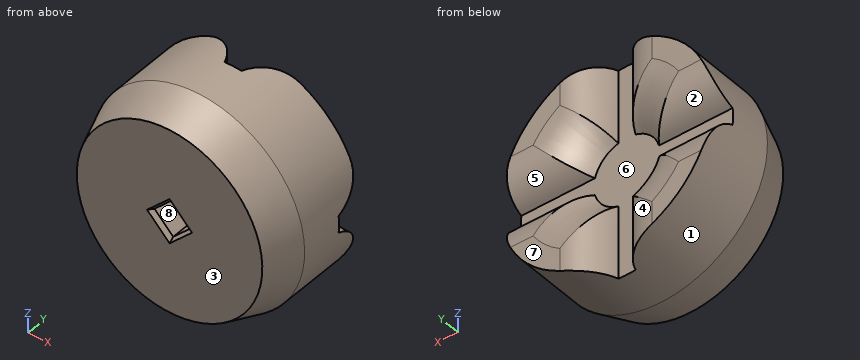
from build123d import *

# Parameters (mm, degrees)
SKETCH3_R           = 8
BOSS_EXTRUDE3_DEPTH = 8
CUT_EXTRUDE2_DEPTH  = 2
CUT_EXTRUDE2_DRAFT  = -10
SKETCH7_R           = 2.5
CUT_EXTRUDE4_DEPTH  = 2
FILLET1_R           = 5
FILLET2_START       = -9
FILLET2_DEPTH       = 18
FILLET2_2_DEPTH     = 18
CUT_EXTRUDE5_DEPTH  = 2.2
CHAMFER2_SIZE       = 0.2
CHAMFER2_SIZE2      = 0.346410162
CHAMFER3_SIZE       = 1
CHAMFER3_SIZE2      = 2.747477419


with BuildPart() as part:
    # Sketch3 → Boss-Extrude3 (new body)
    with BuildSketch(Plane(origin=(0, 0, 0), x_dir=(1, 0, 0), z_dir=(0, 1, 0))):
        with Locations(Location((0, 0, 0), (0, 0, 270))):
            Circle(SKETCH3_R)
    extrude(amount=BOSS_EXTRUDE3_DEPTH)


with BuildPart() as cut_extrude2_tool:
    # Sketch4 → Cut-Extrude2 (with draft: the straight prism first)
    with BuildSketch(Plane(origin=(0, 8, 0), x_dir=(1, 0, 0), z_dir=(0, 1, 0))):
        Polygon((-9, -1), (-1, -1), (-1, -9), (1, -9), (1, -1), (9, -1), (9, 1), (1, 1), (1, 9), (-1, 9), (-1, 1), (-9, 1), align=None)
    extrude(amount=-CUT_EXTRUDE2_DEPTH)
    # Cut-Extrude2: the draft: its side faces are tilted about the plane it starts from
    cut_extrude2_sides = [cut_extrude2_tool.faces().sort_by_distance(p)[0] for p in [
        (-5, 7, 1),
        (-1, 7, 5),
        (0, 7, 9),
        (1, 7, 5),
        (5, 7, 1),
        (9, 7, 0),
        (5, 7, -1),
        (1, 7, -5),
        (0, 7, -9),
        (-1, 7, -5),
        (-5, 7, -1),
        (-9, 7, 0),
    ]]
    draft(cut_extrude2_sides, Plane(origin=(0, 8, 0), x_dir=(1, 0, 0), z_dir=(0, 1, 0)), CUT_EXTRUDE2_DRAFT)


with BuildPart() as part_1:
    add(part.part)

    # Cut-Extrude2: cut by cut_extrude2_tool
    add(cut_extrude2_tool.part, mode=Mode.SUBTRACT)

    # Sketch7 → Cut-Extrude4 (cut)
    with BuildSketch(Plane(origin=(0, 8, 0), x_dir=(1, 0, 0), z_dir=(0, 1, 0))):
        Circle(SKETCH7_R)
    extrude(amount=-CUT_EXTRUDE4_DEPTH, mode=Mode.SUBTRACT)

    # Fillet1
    # the kernel refuses this fillet: 5 mm, written as the material it takes off along each edge
    with BuildSketch(Plane(origin=(0, 8, 0), x_dir=(-0.7093247295722765, 0, -0.7048818539423588), z_dir=(0.7048818539423588, 0, -0.7093247295722765))) as fillet1_piece_1:
        with BuildLine():
            CenterArc((6.5, -5), FILLET1_R, 90, 53.130102354)
            Line((2.5, -2), (2.42, -1.94))
            ThreePointArc((2.42, -1.94), (2.4, -1), (2.4, 0))
            Line((2.4, 0), (2.5, 0.1))
            Line((2.5, 0.1), (6.5, 0.1))
            Line((6.5, 0.1), (6.5, 0))
        make_face()
    revolve(axis=Axis((0, 8, 0), (0, 1, 0)), revolution_arc=359.64, mode=Mode.SUBTRACT)
    with BuildSketch(Plane(origin=(0, 8, 0), x_dir=(0.7048818539423484, 0, -0.7093247295722869), z_dir=(0.7093247295722869, 0, 0.7048818539423484))) as fillet1_piece_2:
        with BuildLine():
            CenterArc((6.5, -5), FILLET1_R, 90, 53.130102354)
            Line((2.5, -2), (2.42, -1.94))
            ThreePointArc((2.42, -1.94), (2.4, -1), (2.4, 0))
            Line((2.4, 0), (2.5, 0.1))
            Line((2.5, 0.1), (6.5, 0.1))
            Line((6.5, 0.1), (6.5, 0))
        make_face()
    revolve(axis=Axis((0, 8, 0), (0, 1, 0)), revolution_arc=359.64, mode=Mode.SUBTRACT)
    with BuildSketch(Plane(origin=(0, 8, 0), x_dir=(0.7093247295722607, 0, 0.7048818539423748), z_dir=(-0.7048818539423748, 0, 0.7093247295722607))) as fillet1_piece_3:
        with BuildLine():
            CenterArc((6.5, -5), FILLET1_R, 90, 53.130102354)
            Line((2.5, -2), (2.42, -1.94))
            ThreePointArc((2.42, -1.94), (2.4, -1), (2.4, 0))
            Line((2.4, 0), (2.5, 0.1))
            Line((2.5, 0.1), (6.5, 0.1))
            Line((6.5, 0.1), (6.5, 0))
        make_face()
    revolve(axis=Axis((0, 8, 0), (0, 1, 0)), revolution_arc=359.64, mode=Mode.SUBTRACT)
    with BuildSketch(Plane(origin=(0, 8, 0), x_dir=(-0.704881853942364, 0, 0.7093247295722713), z_dir=(-0.7093247295722713, 0, -0.704881853942364))) as fillet1_piece_4:
        with BuildLine():
            CenterArc((6.5, -5), FILLET1_R, 90, 53.130102354)
            Line((2.5, -2), (2.42, -1.94))
            ThreePointArc((2.42, -1.94), (2.4, -1), (2.4, 0))
            Line((2.4, 0), (2.5, 0.1))
            Line((2.5, 0.1), (6.5, 0.1))
            Line((6.5, 0.1), (6.5, 0))
        make_face()
    revolve(axis=Axis((0, 8, 0), (0, 1, 0)), revolution_arc=359.64, mode=Mode.SUBTRACT)

    # Fillet2: read off the stored shape, not the designer's step
    # Fillet2 outline → Fillet2 (cut)
    with BuildSketch(Plane.XY.offset(FILLET2_START)):
        with BuildLine():
            ThreePointArc((-3.475773163, 8), (-1.743722356, 7.449489743), (-0.647346039, 6))
            Line((-0.647346039, 6), (-1, 8))
            Line((-1, 8), (-3.475773163, 8))
        make_face()
        with BuildLine():
            Line((1, 8), (0.647346039, 6))
            ThreePointArc((0.647346039, 6), (1.743722356, 7.449489743), (3.475773163, 8))
            Line((3.475773163, 8), (1, 8))
        make_face()
    extrude(amount=FILLET2_DEPTH, mode=Mode.SUBTRACT)

    # Fillet2 2 outline → Fillet2 2 (cut)
    with BuildSketch(Plane.YZ.offset(FILLET2_START)):
        with BuildLine():
            ThreePointArc((8, 3.475773163), (7.449489743, 1.743722356), (6, 0.647346039))
            Line((6, 0.647346039), (8, 1))
            Line((8, 1), (8, 3.475773163))
        make_face()
        with BuildLine():
            Line((8, -1), (6, -0.647346039))
            ThreePointArc((6, -0.647346039), (7.449489743, -1.743722356), (8, -3.475773163))
            Line((8, -3.475773163), (8, -1))
        make_face()
    extrude(amount=FILLET2_2_DEPTH, mode=Mode.SUBTRACT)

    # Sketch5 → Cut-Extrude5 (cut)
    with BuildSketch(Plane.XZ):
        Polygon((1.414213562, 0), (0, -1.414213562), (-1.414213562, 0), (0, 1.414213562), align=None)
    extrude(amount=-CUT_EXTRUDE5_DEPTH, mode=Mode.SUBTRACT)

    # Chamfer2
    chamfer2_edges = [part_1.edges().sort_by_distance(p)[0] for p in [
        (0.7071067811865474, 0, 0.7071067811865479),
        (-0.7071067811865476, 0, 0.7071067811865477),
        (-0.7071067811865474, 0, -0.7071067811865474),
        (0.7071067811865477, 0, -0.7071067811865471),
    ]]
    chamfer2_side = [part_1.faces().sort_by_distance(p)[0] for p in [
        (0, 0, -7.77372583),
    ]]
    chamfer(chamfer2_edges, length=CHAMFER2_SIZE, length2=CHAMFER2_SIZE2, reference=chamfer2_side[0])

    # Chamfer3
    chamfer3_edges = [part_1.edges().sort_by_distance(p)[0] for p in [
        (0, 0, -8),
    ]]
    chamfer3_side = [part_1.faces().sort_by_distance(p)[0] for p in [
        (1.008528137, 0, 1.008528137),
    ]]
    chamfer(chamfer3_edges, length=CHAMFER3_SIZE, length2=CHAMFER3_SIZE2, reference=chamfer3_side[0])


solid = part_1.part
CAD build for the part. Positions are in the model's coordinates, mm. Face numbers are marked on the shaded views. A direction names the side the tool comes from. Round coordinates to 2 decimals unless told otherwise and drop trailing zeros. Write each loop counter-clockwise with the first axis right and the second up, starting at its lowest first coordinate (ties: lowest second). Pieces come first, ordered by that corner, then holes.
(1) Slice it at B-B, the plane y = 0.75. Write the cut outline in (x, z), and give its area (3 significant figures).
(2) Slice it at A-A, the plane y = 7.5. Write the cut outline in (x, z).
(3) 3-axis set-ups, long thin cutter, end or side, ignore diameter. For the marked faces 4, 5, 6, 7 and 8: which of +Z, -Z, +X, -X, +Y, -Y reach the whole face in a straight line?
(4) Mould opens along Z. For the marked faces 1, 2 and 3 say: pulls with the +Z half, pulls with the -Z half, needs draft (parallel to the pull), parting line crosses it, or undercut.
(5) Slice it at C-C, the plane y = 4.5. Write the cut outline in (x, z).
(6) Probe line 1 along Y through (x, z) = (0.25, 1.75); line 2 along Y through (x, z) = (0, -0.5); line 3 along X through (y, z) = (6.75, 6.25). List the from-to ranges inside material, lowest first.
(7) Drop flat-ended pins along their axis: P1, Ø1, axis at x = 2.5, z = 0, coming from the +Y side; P2, Ø3, axis at x = 0.5, y = 6.5, coming from the +Z side; P3, Ø1, axis at y = 1.5, z = 5.5, coming from the -X side; P4, Ø2, axis at x = -6, y = 7, coming from the +Z side (3 decimals). Give the stop position or say it passes through.
From the geometry:
1. outline: circle Ø14.55 at (0, 0); hole (-1.41, 0) - (0, -1.41) - (1.41, 0) - (0, 1.41) - close
1. area: 162 mm2
2. outline: (-7.79, -1.82) arc R8 ccw to (-1.82, -7.79) - (-1.82, -3.92) arc R4.32 cw to (-3.92, -1.82) - close; (-7.79, 1.82) - (-3.92, 1.82) arc R4.32 cw to (-1.82, 3.92) - (-1.82, 7.79) arc R8 ccw to start; (1.82, -7.79) arc R8 ccw to (7.79, -1.82) - (3.92, -1.82) arc R4.32 cw to (1.82, -3.92) - close; (1.82, 3.92) arc R4.32 cw to (3.92, 1.82) - (7.79, 1.82) arc R8 ccw to (1.82, 7.79) - close
3. face 4: +Z, -Z, +Y
3. face 5: +X, -X, +Y
3. face 6: +Y
3. face 7: +Z, -Z, +X, -X, +Y
3. face 8: -Y
4. face 1: parting line crosses it
4. face 2: undercut
4. face 3: needs draft
5. outline: circle Ø16 at (0, 0)
6. line 1: y = 0 to 6
6. line 2: y = 2.2 to 6
6. line 3: x = -4.99 to -1.04, 1.04 to 4.99
7. P1: stops at y = 6
7. P2: stops at z = 8
7. P3: stops at x = -5.71
7. P4: stops at z = 6.245
